```python
from build123d import *

# Parameters (mm, degrees)
FILLET1_R       = 2.5
SKETCH3_W       = 2.16
SKETCH3_H       = 9.8
SKETCH4_W       = 2.16
SKETCH4_H       = 4.175999656
RECPAT_COUNT    = 2
RECPAT_ANGLE    = 90
THDSCHPAT_COUNT = 10
THDSCHPAT_PITCH = 1.5


with BuildPart() as part:
    # BodySke → Base-Revolve (revolve)
    with BuildSketch(Plane.XY):
        Polygon((0, 0), (0, 9.15), (0.85, 9.15), (5, 5), (20, 5), (20, 0), align=None)
    revolve(axis=Axis((-6.35, 0, 0), (1, 0, 0)))

    # Fillet1
    fillet1_edges = [part.edges().sort_by_distance(p)[0] for p in [
        (5, -5, 0),
    ]]
    fillet(fillet1_edges, radius=FILLET1_R)

    # Sketch3 → Recess section 0
    with BuildSketch(Plane.ZY):
        Rectangle(SKETCH3_W, SKETCH3_H)
    # Sketch4 → Recess section 1
    with BuildSketch(Plane.ZY.offset(-5.64)):
        Rectangle(SKETCH4_W, SKETCH4_H)
    recess = loft(mode=Mode.SUBTRACT)

    # RecPat: Recess ×2 about axis
    recpat_axis = Axis((0, 0, 0), (1, 0, 0))
    for i in range(1, RECPAT_COUNT):
        add(recess.rotate(recpat_axis, i * RECPAT_ANGLE / (RECPAT_COUNT - 1)), mode=Mode.SUBTRACT)

    # RecCorSke → RecessCore (revolve, cut)
    with BuildSketch(Plane.XY):
        Polygon((0, 0), (0, 2.324887219), (5.64, 1.9305), (6.267257474, 0), align=None)
    revolve(axis=Axis((-3.175, 0, 0), (1, 0, 0)), mode=Mode.SUBTRACT)

    # ThdSchSke → ThreadSchematic (revolve, cut)
    with BuildSketch(Plane.XY):
        Polygon((6.500001, -4.172), (5.920229158, -5), (5.920229158, -6.25), (7.079772842, -6.25), (7.079772842, -5), align=None)
    threadschematic = revolve(axis=Axis((-3.175, 0, 0), (1, 0, 0)), mode=Mode.SUBTRACT)

    # ThdSchPat: ThreadSchematic ×10
    with Locations(*[(i * THDSCHPAT_PITCH, 0, 0) for i in range(1, THDSCHPAT_COUNT)]):
        add(threadschematic, mode=Mode.SUBTRACT)


solid = part.part
```
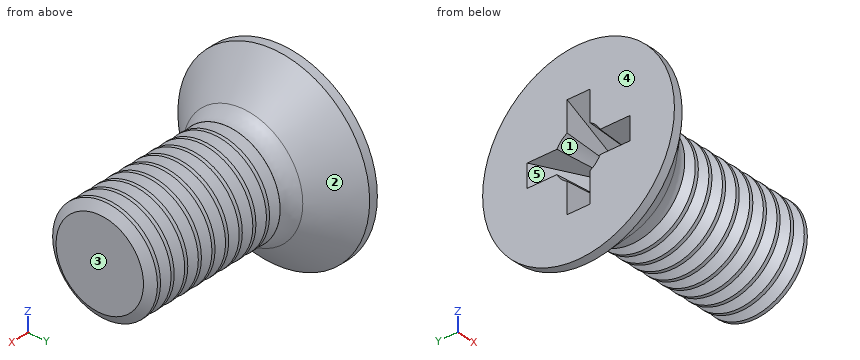
Geometry check sheet. Reference: the model listing, model coordinates, mm. Face numbers are marked on the shaded views. A direction names the side the tool comes from. Give positions to 0.01 mm unless a question says otherwise; leave off trailing zeros. One line per question, with ' | ' between items.
Item 1: Depth check by flat-ended pin: pin 1 (3 mm diameter, centred on x = 15, z = 5.5, fed in from +Y); pin 2 (8 mm diameter, centred on x = 5, y = 3, fed in from +Z); pin 3 (10 mm diameter, centred on x = 12, y = 6.5, fed in from -Z). Enter the tip coordinate at first touch or a pass-through.
Determined:
pin 1: y = 3 | pin 2: z = 8.65 | pin 3: z = -4.77
Item 2: Scan lines: line 1 along Z through (x, y) = (1.75, -1); line 2 along Y through (x, z) = (2, -1); line 3 along Y through (x, z) = (4.5, 1.25). Record each from-to range of solid material in increasing order.
Determined:
line 1: -8.19 to -4.03, 4.03 to 8.19 | line 2: -7.94 to -3.9, 3.9 to 7.94 | line 3: -5.38 to -1.57, 1.57 to 5.38
Item 3: Draft check along Y on the marked faces 1, 2 and 3. Enter one of: released by +Y, released by -Y, zero draft, split by the parting line, or undercut.
Determined:
face 1: undercut | face 2: split by the parting line | face 3: zero draft
Item 4: Sectioned sample at A-A, the plane y = 4.5. State how many separate pieces and enclosed holes the cut face has, plus the area to 3 significant figures.
Determined:
separate pieces: 10 | enclosed holes: 0 | area: 93.3 mm^2
Item 5: Access from +Z, -Z, +X, -X, +Y, -Y to the whole of each face (thin tool, end or side, straight path). Record for the marked faces 4 and 5.
Determined:
face 4: +Z, -Z, -X, +Y, -Y | face 5: -X
